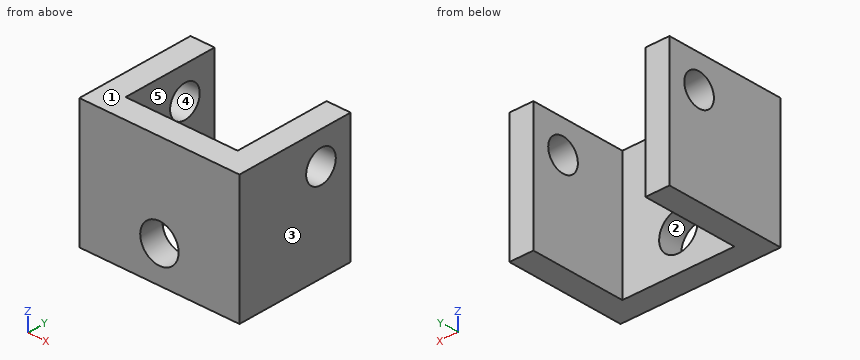
from build123d import *

# Parameters (mm, degrees)
SKETCH1_W           = 10
SKETCH1_H           = 8
BOSS_EXTRUDE1_DEPTH = 1.5
SKETCH3_W           = 1.5
SKETCH3_H           = 8
BOSS_EXTRUDE2_DEPTH = 6
SKETCH4_R           = 1.2
CUT_EXTRUDE1_DEPTH  = 9.774964387
SKETCH5_R           = 1
CUT_EXTRUDE2_DEPTH  = 14.124404748


with BuildPart() as part:
    # Sketch1 → Boss-Extrude1 (new body)
    with BuildSketch(Plane(origin=(0, 0, 0), x_dir=(1, 0, 0), z_dir=(0, 1, 0))):
        Rectangle(SKETCH1_W, SKETCH1_H)
    extrude(amount=BOSS_EXTRUDE1_DEPTH)

    # Sketch3 → Boss-Extrude2 (add)
    with BuildSketch(Plane(origin=(0, 1.5, 0), x_dir=(1, 0, 0), z_dir=(0, 1, 0))):
        with Locations((-4.25, 0)):
            Rectangle(SKETCH3_W, SKETCH3_H)
        with Locations((4.25, 0)):
            Rectangle(SKETCH3_W, SKETCH3_H)
    extrude(amount=BOSS_EXTRUDE2_DEPTH)

    # Sketch4 → Cut-Extrude1 (cut, through all)
    with BuildSketch(Plane(origin=(0, 1.5, 0), x_dir=(1, 0, 0), z_dir=(0, 1, 0))):
        with Locations(Location((0, 1.734711092, 0), (0, 0, 270))):
            Circle(SKETCH4_R)
    extrude(amount=-CUT_EXTRUDE1_DEPTH, mode=Mode.SUBTRACT)

    # Sketch5 → Cut-Extrude2 (cut, through all)
    with BuildSketch(Plane.ZY.offset(5)):
        with Locations((2, 5.5)):
            Circle(SKETCH5_R)
    extrude(amount=-CUT_EXTRUDE2_DEPTH, mode=Mode.SUBTRACT)


solid = part.part
Verification items for the finished model (mm, model axes). Face numbers are marked on the shaded views. A direction names the side the tool comes from. Give positions to 0.01 mm unless a question says otherwise; leave off trailing zeros. Write each loop counter-clockwise with the first axis right and the second up, starting at its lowest first coordinate (ties: lowest second). Pieces come first, ordered by that corner, then holes. Notation, with made-up numbers: (84.25, 69) -> (123.25, 69) arc R25 cw to (123.25, 102) -> close; hole circle Ø11 at (67.25, 36.5). An arc over 180 degrees is marked (long way). Use CSV: the item, a comma, the result in double quotes.
(1) Sectioned sample at B-B (z = 2). Record the cut outline in (x, y), plus the area to 3 significant figures.
Derived:
outline,"(-5, 0) -> (5, 0) -> (5, 4.5) -> (3.5, 4.5) -> (3.5, 1.5) -> (-3.5, 1.5) -> (-3.5, 4.5) -> (-5, 4.5) -> close; (-5, 6.5) -> (-3.5, 6.5) -> (-3.5, 7.5) -> (-5, 7.5) -> close; (3.5, 6.5) -> (5, 6.5) -> (5, 7.5) -> (3.5, 7.5) -> close"
area,"27.0 mm^2"
(2) Sectioned sample at C-C (x = 0). Record the cut outline in (y, z).
Derived:
outline,"(0, -4) -> (1.5, -4) -> (1.5, -2.93) -> (0, -2.93) -> close; (0, -0.53) -> (1.5, -0.53) -> (1.5, 4) -> (0, 4) -> close"
(3) Sectioned sample at A-A (y = 5.5). Record the cut outline in (x, z).
Derived:
outline,"(-5, -4) -> (-3.5, -4) -> (-3.5, 1) -> (-5, 1) -> close; (-5, 3) -> (-3.5, 3) -> (-3.5, 4) -> (-5, 4) -> close; (3.5, -4) -> (5, -4) -> (5, 1) -> (3.5, 1) -> close; (3.5, 3) -> (5, 3) -> (5, 4) -> (3.5, 4) -> close"
(4) Material ranges on L1, parallel to X at y = 3.75, z = -2.75; L2, parallel to Y at x = -3.8, z = 2; L3, parallel to Y at x = 2, z = -2.5, recorded low to high.
Derived:
L1,"x = -5 to -3.5, 3.5 to 5"
L2,"y = 0 to 4.5, 6.5 to 7.5"
L3,"y = 0 to 1.5"
(5) Go/stop test with flat-tipped pins: pin 1 (2 mm diameter, centred on x = 1, z = -0.5, fed in from +Y); pin 2 (1.6 mm diameter, centred on y = 5.5, z = 2, fed in from +X). Record where each tip stops, or that it passes through.
Derived:
pin 1,"stops at y = 1.5"
pin 2,"passes through"
(6) Sectioned sample at D-D (y = 2.5). Record the cut outline in (x, z).
Derived:
outline,"(-5, -4) -> (-3.5, -4) -> (-3.5, 4) -> (-5, 4) -> close; (3.5, -4) -> (5, -4) -> (5, 4) -> (3.5, 4) -> close"
(7) Release check for a two-part mould opening along X. For the marked faces 1, 2 and 3 record: +X half, -X half, draft (parallel to the pull), parting line (faces both ways), or undercut.
Derived:
face 1,"draft"
face 2,"undercut"
face 3,"+X half"
(8) Set-up check for the marked faces 4 and 5: record each of +Z, -Z, +X, -X, +Y, -Y from which the full face is reachable in a straight line by a thin tool's end or side.
Derived:
face 4,"+X, -X"
face 5,"+Z, -Z, +Y"
